Can you work these out from the drawing? Everything is in mm from the part's minimum corner. A direction names the side the tool comes from. Give positions to 0.01 mm unless a question says otherwise; leave off trailing zeros. Write each loop counter-clockwise with the first axis right and the second up, starting at its lowest first coordinate (ties: lowest second). Pieces come first, ordered by that corner, then holes. Notation, with made-up numbers: (78, 7.25) -> (107, 7.25) arc R20 cw to (107, 30.25) -> close; hole circle Ø11 at (17.5, 6.5). An arc over 180 degrees is marked (long way). Use one line per item in the form item = value.
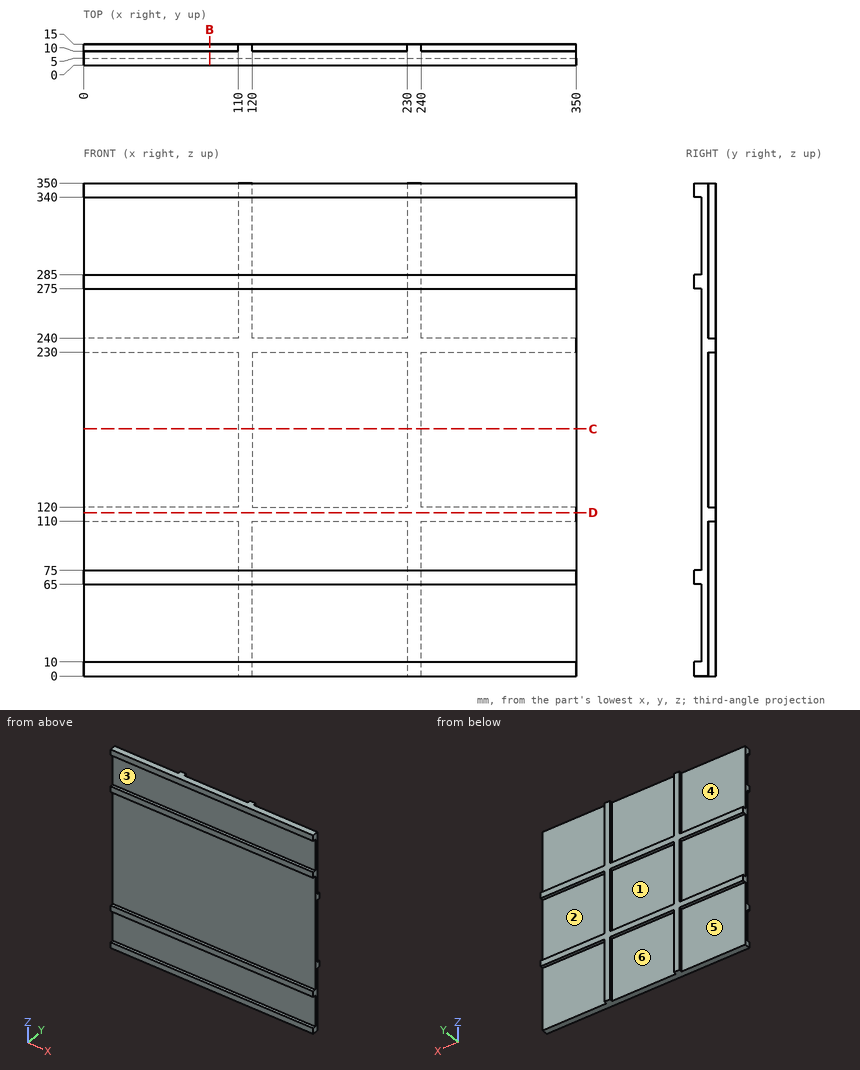
Q1. If I drill on line 1 along Z through (x, y) = (307.5, 2.5); line 2 along Z through (x, y) = (57, 13), over which ranges is the centre line in solid material (lowest first)? Write a range as from..to.
Result set:
line_1 = 0..10, 65..75, 275..285, 340..350
line_2 = 110..120, 230..240
Q2. Will these pins go through, and if not, where does the flat tip stop? pin 1 Ø1.5 at (y, z) = (13.5, 319.5) entering from +X; pin 2 Ø4 at (x, z) = (72, 281) entering from +Y; pin 3 Ø16.5 at (x, z) = (156, 318) entering from -Y.
Result set:
pin_1 = 240
pin_2 = 10
pin_3 = 5
Q3. I want a section at C-C, the plane z = 175.5. Write out the boundary of the cut face in (x, y).
Result set:
outline = (0, 5) -> (350, 5) -> (350, 10) -> (240, 10) -> (240, 15) -> (230, 15) -> (230, 10) -> (120, 10) -> (120, 15) -> (110, 15) -> (110, 10) -> (0, 10) -> close
Q4. I want a section at B-B, the plane x = 89.5. Write out the boundary of the cut face in (y, z).
Result set:
outline = (0, 0) -> (10, 0) -> (10, 110) -> (15, 110) -> (15, 120) -> (10, 120) -> (10, 230) -> (15, 230) -> (15, 240) -> (10, 240) -> (10, 350) -> (0, 350) -> (0, 340) -> (5, 340) -> (5, 285) -> (0, 285) -> (0, 275) -> (5, 275) -> (5, 75) -> (0, 75) -> (0, 65) -> (5, 65) -> (5, 10) -> (0, 10) -> close
Q5. If we mould it in two halves opening along X, with no side actions, what happens to the marked faces 5 and 6? For each: +X half, -X half, draft (parallel to the pull), parting line (faces both ways), or undercut.
Result set:
face_5 = draft
face_6 = undercut
Q6. I want a section at D-D, the plane z = 116. Write out the boundary of the cut face in (x, y), and give its area (3 significant figures).
Result set:
outline = (0, 5) -> (350, 5) -> (350, 15) -> (0, 15) -> close
area = 3,500 mm2
Q7. Which directions (+Z, -Z, +X, -X, +Y, -Y) give clear straight access to the entire face, cutting with the end or side of a thin tool? Please do the marked faces 1, 2, 3 and 4.
Result set:
face_1 = +Y
face_2 = +X, +Y
face_3 = +X, -X, -Y
face_4 = +Z, -X, +Y
